Work out the finished part from the listing and answer in its coordinate system (mm). A direction names the side the tool comes from. Round coordinates to 2 decimals unless told otherwise and drop trailing zeros. Write each loop counter-clockwise with the first axis right and the second up, starting at its lowest first coordinate (ties: lowest second). Pieces come first, ordered by that corner, then holes.
1. Find section B-B (z = -3.5). Write down the section's boundary in (x, y), and give its area (3 significant figures).
2. Find section A-A (x = -3.75). Write down the section's boundary in (y, z), and give its area (3 significant figures).
3. Straight lines are drawn through the part: probe 1 along X at (y, z) = (-74.5, 13); probe 2 along Y at (x, z) = (10.25, 3); probe 3 along Z at (x, y) = (11.75, -41.5). For each, find the intervals that lie inside material, in ascending order.
4. Determine the mould class of faces 1 (the face through (2, 2, -12.659)), 2 (the face through (-9.852, 2, -9)), 3 (the face through (6.148, 2, 13)) for opening direction Z: pulls with the +Z half, pulls with the -Z half, needs draft (parallel to the pull), parting line crosses it, or undercut.
5. Find section D-D (y = -68). Write down the section's boundary in (x, z).
6. Flat-ended cylindrical pins translate along their axes: pin 1 Ø4 at (x, z) = (0, -8) entering from -Y; pin 2 Ø11.5 at (y, z) = (-23.5, 2) entering from -X; pin 3 Ø3 at (x, y) = (13, -42) entering from +Z. Find the tip coordinate at first contact, or state that the pin passes through.
7. A tool of negligible diameter and unlimited length cuts with its end or side. For faces 4 (the face through (13, -39, 16.341)), 5 (the face through (-2, 2, -1.159)), 6 (the face through (13, -39, -6.659)), from which of +Z, -Z, +X, -X, +Y, -Y can it reach the whole face along a straight path? Write none if from no direction.
8. Find section C-C (x = 7). Write down the section's boundary in (y, z).
```python
from build123d import *

# Parameters (mm, degrees)
SKETCH1_W           = 25
SKETCH1_H           = 35
BOSS_EXTRUDE1_DEPTH = 4
SKETCH2_W           = 16
SKETCH2_H           = 4.5
CUT_EXTRUDE1_DEPTH  = 4
SKETCH3_W           = 3.5
SKETCH3_H           = 23
BOSS_EXTRUDE2_DEPTH = 80


with BuildPart() as part:
    # Sketch1 → Boss-Extrude1 (new body)
    with BuildSketch(Plane(origin=(0, 0, 0), x_dir=(1, 0, 0), z_dir=(0, 1, 0))):
        with Locations((2.648305085, -4.841101695)):
            Rectangle(SKETCH1_W, SKETCH1_H)
    extrude(amount=BOSS_EXTRUDE1_DEPTH)

    # Sketch2 → Cut-Extrude1 (cut)
    with BuildSketch(Plane(origin=(0, 4, 0), x_dir=(1, 0, 0), z_dir=(0, 1, 0))):
        with Locations((-1.851694915, -13.091101695)):
            Rectangle(SKETCH2_W, SKETCH2_H)
        with Locations((-1.851694915, 3.408898305)):
            Rectangle(SKETCH2_W, SKETCH2_H)
    extrude(amount=-CUT_EXTRUDE1_DEPTH, mode=Mode.SUBTRACT)

    # Sketch3 → Boss-Extrude2 (add)
    with BuildSketch(Plane(origin=(0, 0, 0), x_dir=(-1, 0, 0), z_dir=(0, -1, 0))):
        with Locations((-13.398305085, -4.841101695)):
            Rectangle(SKETCH3_W, SKETCH3_H)
    extrude(amount=BOSS_EXTRUDE2_DEPTH)


solid = part.part
```
Worked answers:
1. outline: (6.15, 0) - (11.65, 0) - (11.65, -80) - (15.15, -80) - (15.15, 4) - (6.15, 4) - close
1. area: 316 mm2
2. outline: (0, -12.66) - (4, -12.66) - (4, -5.66) - (0, -5.66) - close; (0, -1.16) - (4, -1.16) - (4, 10.84) - (0, 10.84) - close; (0, 15.34) - (4, 15.34) - (4, 22.34) - (0, 22.34) - close
2. area: 104 mm2
3. probe 1: x = 11.65 to 15.15
3. probe 2: y = 0 to 4
3. probe 3: z = -6.66 to 16.34
4. face 1: pulls with the -Z half
4. face 2: needs draft
4. face 3: undercut
5. outline: (11.65, -6.66) - (15.15, -6.66) - (15.15, 16.34) - (11.65, 16.34) - close
6. pin 1: stops at y = 0
6. pin 2: stops at x = 11.65
6. pin 3: stops at z = 16.34
7. face 4: +Z, +X, -X, -Y
7. face 5: -X, +Y, -Y
7. face 6: -Z, +X, -X, -Y
8. outline: (0, -12.66) - (4, -12.66) - (4, 22.34) - (0, 22.34) - close
